For this review, take the finished solid that the model builds, in its own axes (mm). A direction names the side the tool comes from. Round coordinates to 2 decimals unless told otherwise and drop trailing zeros. Order: outer loops, then holes, each group sorted by start corner. A loop starts at its lowest first (then second) coordinate and runs counter-clockwise, first axis right, second up. Notation, with made-up numbers: M -9.75,51.25 L 3.25,51.25 A19 ccw 3.25,59.25 Z; hole C 72.25,-25.75 d7. An arc over 180 degrees is marked long. Answer as a JSON object with one key per item and string values.
from build123d import *

# Parameters (mm, degrees)
F0_W     = 628.65
F0_H     = 19.05
F1_DEPTH = 711.2
F2_W     = 330.2
F2_H     = 101.6
F2_H_2   = 127
F3_DEPTH = 25.4


with BuildPart() as f1:
    # F0 (on Front) → F1 (new body)
    with BuildSketch(Plane.XZ):
        Rectangle(F0_W, F0_H)
    extrude(amount=F1_DEPTH)

    # F2 (on face) → F3 (cut)
    with BuildSketch(Plane.XY.offset(9.525)):
        with Locations((0, -203.2)):
            Rectangle(F2_W, F2_H)
        with Locations((0, -355.6)):
            Rectangle(F2_W, F2_H)
        with Locations((0, -596.9)):
            Rectangle(F2_W, F2_H_2)
    extrude(amount=-F3_DEPTH, mode=Mode.SUBTRACT)


solid = f1.part
1) Mouldability with a two-part tool opening along Y and no side actions: class faces 3 (the flat face through (165.1, -204, 0)), 4 (the flat face through (314.325, -351, 0)), 5 (the flat face through (-4, -711.2, 0)) as +Y half, -Y half, draft (parallel to the pull), parting line (faces both ways), or undercut.
Geometry check:
{"face 3": "undercut", "face 4": "draft", "face 5": "-Y half"}
2) Add section C-C on y = -626. State the section outline as (x, z) points (3 decimals).
Geometry check:
{"outline": "M -314.325,-9.525 L -165.1,-9.525 L -165.1,9.525 L -314.325,9.525 Z; M 165.1,-9.525 L 314.325,-9.525 L 314.325,9.525 L 165.1,9.525 Z"}
3) Add section B-B on z = -2.75. State the section outline as (x, y) points (3 decimals), and give its area (3 significant figures).
Geometry check:
{"outline": "M -314.325,-711.2 L 314.325,-711.2 L 314.325,0 L -314.325,0 Z; hole M -165.1,-660.4 L 165.1,-660.4 L 165.1,-533.4 L -165.1,-533.4 Z; hole M -165.1,-406.4 L 165.1,-406.4 L 165.1,-304.8 L -165.1,-304.8 Z; hole M -165.1,-254 L 165.1,-254 L 165.1,-152.4 L -165.1,-152.4 Z", "area": "338,000 mm²"}
4) For L1, parallel to Y at x = -90, z = 6.5; L2, parallel to X at y = -607, z = -8.25 (3 decimals), list the stretches that pass through material, from the lowest coordinate up.
Geometry check:
{"L1": "y = -711.2 to -660.4, -533.4 to -406.4, -304.8 to -254, -152.4 to 0", "L2": "x = -314.325 to -165.1, 165.1 to 314.325"}
5) Insertion check: P1, Ø9.5, axis at x = -41.5, z = 4, coming from the +Y side. The pin has a flat end and moves straight along its axis. Give the tip position at first contact, or say it passes through.
Geometry check:
{"P1": "stops at y = 0"}
6) Machinability: for faces 1 (the flat face through (-4, -272, -9.525)), 2 (the flat face through (-2, -406.4, 0)), which of the approach directions +Z, -Z, +X, -X, +Y, -Y give a long, thin tool a straight path to every point of the face, cutting with its end or side? Answer none if there is none.
Geometry check:
{"face 1": "-Z, +X, -X, +Y, -Y", "face 2": "+Z, -Z"}
7) Add section A-A on x = 42. State the section outline as (y, z) points (3 decimals).
Geometry check:
{"outline": "M -711.2,-9.525 L -660.4,-9.525 L -660.4,9.525 L -711.2,9.525 Z; M -533.4,-9.525 L -406.4,-9.525 L -406.4,9.525 L -533.4,9.525 Z; M -304.8,-9.525 L -254,-9.525 L -254,9.525 L -304.8,9.525 Z; M -152.4,-9.525 L 0,-9.525 L 0,9.525 L -152.4,9.525 Z"}
